The listing builds one solid part. Answer for the finished solid, in the listing's coordinates (mm). Face numbers are marked on the shaded views. A direction names the side the tool comes from. Round coordinates to 2 decimals unless told otherwise and drop trailing zeros. Order: outer loops, then holes, each group sorted by start corner. A loop starts at its lowest first (then second) coordinate and runs counter-clockwise, first axis right, second up. Notation, with made-up numbers: (9.25, 85) - (64.25, 85) arc R16 ccw to (64.25, 105) - close; hole circle Ø8 at (-27, 61). An arc over 180 degrees is marked (long way). One line per item, written item: value. Start each with the question number.
1. Straight lines are drawn through the part: line 1 (Z direction, x = -51, y = 88); line 2 (Y direction, x = 54, z = 48); line 3 (Z direction, x = 43.5, y = 100.5). For each, find the intervals that lie inside material, in ascending order.
2. For a pull along X with two mould halves and no side action, classify the marked faces 4, 5 and 6 as released by +X, released by -X, zero draft, split by the parting line, or undercut.
3. A tool of negligible diameter and unlimited length cuts with its end or side. For the marked faces 1, 2 and 3, from which of +Z, -Z, +X, -X, +Y, -Y can it reach the whole face along a straight path? Write none if from no direction.
4. Flat-ended cylindrical pins translate along their axes: P1, Ø1, axis at x = -39.5, z = -50.5, coming from the -Y side; P2, Ø10, axis at x = -73, z = -64.5, coming from the -Y side; P3, Ø10, axis at x = 45.5, y = 161.5, coming from the -Z side; P4, Ø1, axis at y = 75.5, z = 50, coming from the +X side. Find the tip coordinate at first contact, or state that the pin passes through.
5. Section A-A, the plane x = -18.5 is taken. Give the vertices of the cut face in (y, z).
6. Section B-B, the plane x = -46.5 is taken. Give the vertices of the cut face in (y, z), then the cut area to 3 significant figures.
from build123d import *

# Parameters (mm, degrees)
BOSS_EXTRUDE3_DEPTH = 20


with BuildPart() as part:
    # Sketch1 → Revolve-Thin2 (revolve)
    with BuildSketch(Plane.XY):
        Polygon((29.376248058, -59.973392874), (0.560391904, -35.876681975), (-24.659832096, -60.795812358), (-65.01956382, -27.045755372), (-65.01956382, 32.372412999), (65.01956382, 32.372412999), (65.01956382, -26.719075047), align=None)
        Polygon((29.014074927, -46.634880572), (0, -22.372412999), (-25.220224001, -47.291543383), (-55.01956382, -22.372412999), (-55.01956382, 22.372412999), (55.01956382, 22.372412999), (55.01956382, -22.372412999), align=None, mode=Mode.SUBTRACT)
    revolve(axis=Axis((-55.01956382, 84.277813771, 0), (1, 0, 0)))

    # Sketch2 → Boss-Extrude3 (add)
    with BuildSketch(Plane.ZY.offset(65.01956382)):
        with BuildLine():
            Line((-51.905400772, 84.277813771), (-76.712133876, 84.277813771))
            Line((-76.712133876, 84.277813771), (-74.341443656, 89.433234307))
            ThreePointArc((-74.341443656, 89.433234307), (-60.775134761, 106.881443528), (-40.875379676, 116.498329179))
            Line((-40.875379676, 116.498329179), (-40.654960426, 116.547688609))
            Line((-40.654960426, 116.547688609), (-45.427875958, 109.387148992))
            Line((-45.427875958, 109.387148992), (-49.616909483, 99.520284788))
            Line((-49.616909483, 99.520284788), (-51.648739272, 89.433234307))
            Line((-51.648739272, 89.433234307), (-51.905400772, 84.277813771))
        make_face()
        with BuildLine():
            Line((-25.952700386, 129.229209434), (-38.356066938, 150.712470486))
            Line((-38.356066938, 150.712470486), (-32.705996677, 151.2371028))
            ThreePointArc((-32.705996677, 151.2371028), (-10.812249793, 148.212439271), (7.466095028, 135.787188664))
            Line((7.466095028, 135.787188664), (7.619051174, 135.620979709))
            Line((7.619051174, 135.620979709), (-0.968615806, 136.174176002))
            Line((-0.968615806, 136.174176002), (-11.608087624, 134.868553349))
            Line((-11.608087624, 134.868553349), (-21.359644485, 131.584644322))
            Line((-21.359644485, 131.584644322), (-25.952700386, 129.229209434))
        make_face()
        with BuildLine():
            Line((25.952700386, 129.229209434), (38.356066938, 150.712470486))
            Line((38.356066938, 150.712470486), (41.635446979, 146.081682264))
            ThreePointArc((41.635446979, 146.081682264), (49.962884968, 125.608809514), (48.341474704, 103.566673256))
            Line((48.341474704, 103.566673256), (48.2740116, 103.351104871))
            Line((48.2740116, 103.351104871), (44.459260153, 111.064840781))
            Line((44.459260153, 111.064840781), (38.008821859, 119.626082332))
            Line((38.008821859, 119.626082332), (30.289094787, 126.429223787))
            Line((30.289094787, 126.429223787), (25.952700386, 129.229209434))
        make_face()
        with BuildLine():
            Line((51.905400772, 84.277813771), (76.712133876, 84.277813771))
            Line((76.712133876, 84.277813771), (74.341443656, 79.122393235))
            ThreePointArc((74.341443656, 79.122393235), (60.775134761, 61.674184014), (40.875379676, 52.057298364))
            Line((40.875379676, 52.057298364), (40.654960426, 52.007938933))
            Line((40.654960426, 52.007938933), (45.427875958, 59.16847855))
            Line((45.427875958, 59.16847855), (49.616909483, 69.035342754))
            Line((49.616909483, 69.035342754), (51.648739272, 79.122393235))
            Line((51.648739272, 79.122393235), (51.905400772, 84.277813771))
        make_face()
        with BuildLine():
            Line((25.952700386, 39.326418109), (38.356066938, 17.843157056))
            Line((38.356066938, 17.843157056), (32.705996677, 17.318524743))
            ThreePointArc((32.705996677, 17.318524743), (10.812249793, 20.343188271), (-7.466095028, 32.768438879))
            Line((-7.466095028, 32.768438879), (-7.619051174, 32.934647833))
            Line((-7.619051174, 32.934647833), (0.968615806, 32.381451541))
            Line((0.968615806, 32.381451541), (11.608087624, 33.687074193))
            Line((11.608087624, 33.687074193), (21.359644485, 36.97098322))
            Line((21.359644485, 36.97098322), (25.952700386, 39.326418109))
        make_face()
        with BuildLine():
            Line((-25.952700386, 39.326418109), (-38.356066938, 17.843157056))
            Line((-38.356066938, 17.843157056), (-41.635446979, 22.473945279))
            ThreePointArc((-41.635446979, 22.473945279), (-49.962884968, 42.946818028), (-48.341474704, 64.988954286))
            Line((-48.341474704, 64.988954286), (-48.2740116, 65.204522671))
            Line((-48.2740116, 65.204522671), (-44.459260153, 57.490786762))
            Line((-44.459260153, 57.490786762), (-38.008821859, 48.929545211))
            Line((-38.008821859, 48.929545211), (-30.289094787, 42.126403756))
            Line((-30.289094787, 42.126403756), (-25.952700386, 39.326418109))
        make_face()
    extrude(amount=BOSS_EXTRUDE3_DEPTH)


solid = part.part
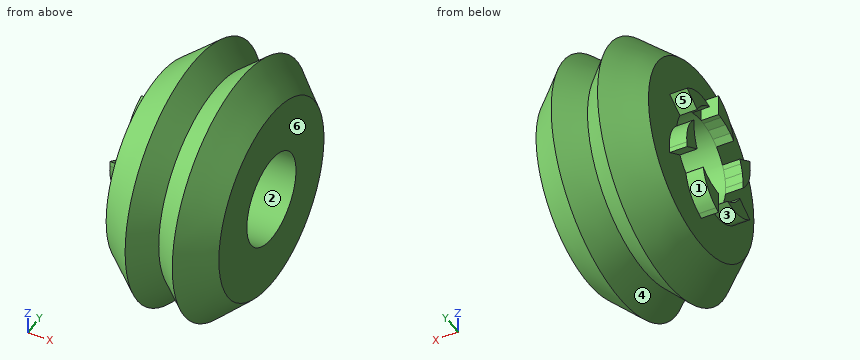
Answer list:
1. line 1: z = -122.99 to -109.95, -61.79 to -51.77, 51.77 to 61.79, 109.95 to 122.99
1. line 2: y = -27.1 to -12.02, 45.18 to 64.53, 104.03 to 123.37, 180.58 to 195.65
1. line 3: z = -130.07 to -116.27, -59.74 to -49.31, 49.31 to 59.74, 116.27 to 130.07
2. face 4: undercut
2. face 5: zero draft
2. face 6: released by +X
3. face 1: -Z, -X, +Y
3. face 2: +X
3. face 3: -Z, -X
4. P1: stops at y = -38.89
4. P2: stops at y = 84.28
4. P3: stops at z = -110.33
4. P4: passes through
5. outline: circle Ø277.97 at (84.28, 0); circle Ø123.81 at (84.28, 0); hole circle Ø249.86 at (84.28, 0); hole circle Ø103.81 at (84.28, 0)
6. outline: circle Ø253.62 at (84.28, 0); circle Ø123.81 at (84.28, 0); hole circle Ø227.55 at (84.28, 0); hole circle Ø103.81 at (84.28, 0)
6. area: 13,400 mm²
